Build history of the part. All positions in model axes, mm. Face numbers are marked on the shaded views. Coordinates: 2 decimals unless noted, no trailing zeros. Write each loop counter-clockwise with the first axis right and the second up, starting at its lowest first coordinate (ties: lowest second). Pieces come first, ordered by that corner, then holes.
from build123d import *

# Parameters (mm, degrees)
F0_R     = 41.5
F1_DEPTH = 90
F2_R     = 37.351414
F3_DEPTH = 80
F4_R     = 3


with BuildPart() as f1:
    # F0 (on Top) → F1 (new body)
    with BuildSketch(Plane.XY):
        Circle(F0_R)
    extrude(amount=-F1_DEPTH)

    # F2 (on face) → F3 (cut)
    with BuildSketch(Plane.XY):
        Circle(F2_R)
    extrude(amount=-F3_DEPTH, mode=Mode.SUBTRACT)

    # F4
    f4_edges = [f1.edges().sort_by_distance(p)[0] for p in [
        (41.5, 0, -45),
        (-41.5, 0, 0),
        (-41.5, 0, -90),
    ]]
    fillet(f4_edges, radius=F4_R)


solid = f1.part
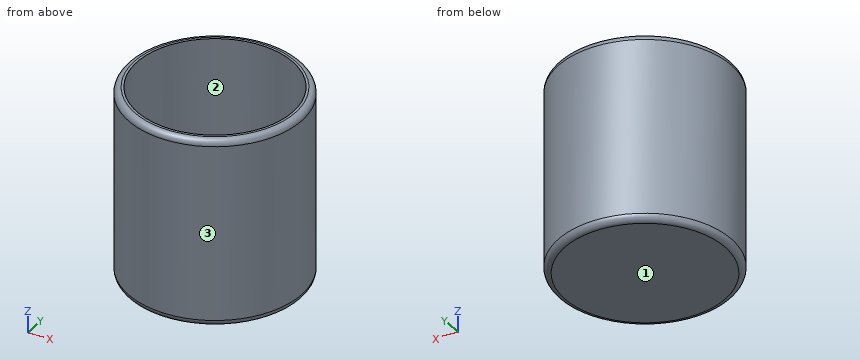
(1) Slice it at A-A, the plane x = 0. List the corners of the cut face in (y, z), and give its area (3 significant figures).
(2) Probe L1, parallel to Y at x = 0, z = -50; L2, parallel to Z at x = -3.5, y = 25; L3, parallel to Y at x = 13.5, z = -11. List the from-to ranges inside material, lowest first.
(3) Slice it at C-C, the plane z = -58.5. List the corners of the cut face in (x, y).
(4) Flat gauge pins, fed straight in: P1, Ø1, axis at x = 1.5, y = 22.5, coming from the +Z side; P2, Ø12, axis at y = -30.5, z = -72.5, coming from the -X side; P3, Ø3, axis at x = -8.5, z = -60, coming from the -Y side. Where does each tip first touch, or does it go through?
(5) Two-plate mould, pull along Y, no slides. Class the marked faces 1, 2 and 3: pulls with the +Y half, pulls with the -Y half, needs draft (parallel to the pull), parting line crosses it, or undercut.
Results:
1. outline: (-41.5, -87) arc R3 ccw to (-38.5, -90) - (38.5, -90) arc R3 ccw to (41.5, -87) - (41.5, -3) arc R3 ccw to (38.5, 0) - (37.35, 0) - (37.35, -80) - (-37.35, -80) - (-37.35, 0) - (-38.5, 0) arc R3 ccw to (-41.5, -3) - close
1. area: 1,490 mm2
2. L1: y = -41.5 to -37.35, 37.35 to 41.5
2. L2: z = -90 to -80
2. L3: y = -39.24 to -34.83, 34.83 to 39.24
3. outline: circle Ø83 at (0, 0); hole circle Ø74.7 at (0, 0)
4. P1: stops at z = -80
4. P2: stops at x = -33.5
4. P3: stops at y = -40.91
5. face 1: needs draft
5. face 2: undercut
5. face 3: parting line crosses it
